Verification items for the finished model (mm, model axes). A direction names the side the tool comes from. Coordinates: 2 decimals unless noted, no trailing zeros. Loops run counter-clockwise (first coordinate to the right, second up) from the corner with the lowest first, then second, coordinate; pieces in that order, holes last. Notation, with made-up numbers: (-8.75, 37.5) - (5.25, 37.5) arc R19 ccw to (5.25, 72.5) - close; hole circle Ø8 at (68, 60.25). An arc over 180 degrees is marked (long way). One line per item, written item: value. Start each with the question number.
(1) Draft check along Z on faces 6 (the face through (18, -20, 0)), 7 (the face through (6, -64, 7)), 8 (the face through (16, -63, 0.3)), 9 (the face through (5, -69, 14)). Enter one of: +Z half, -Z half, draft (parallel to the pull), parting line (faces both ways), or undercut.
(2) Section check A-A (z = 14). Record the boundary of the cut face in (x, y).
(3) Set-up check for faces 1 (the face through (13.594, -40.048, 5.67)), 2 (the face through (5, -69, 4)), 3 (the face through (19, -21, 11.5)), 4 (the face through (9, -10, 6)), 5 (the face through (2.24, -10.52, 0.15)): record each of +Z, -Z, +X, -X, +Y, -Y from which the full face is reachable in a straight line by a thin tool's end or side.
(4) Section check C-C (z = 4). Record the boundary of the cut face in (x, y), plus the area to 3 significant figures.
(5) Section check D-D (y = -3.8). Record the boundary of the cut face in (x, z).
(6) Thickness scan on probe 1 along Z at (x, y) = (4, -70); probe 2 along Z at (x, y) = (1, 6.5); probe 3 along Y at (x, z) = (4.3, 14). Record the ranges inside material, lowest first. Write a range as [from, to].
(7) Section check B-B (x = 20.5). Record the boundary of the cut face in (y, z), plus the area to 3 significant figures.
(8) Gauge pin test, flat ends, axial feed: P1, Ø4, axis at y = 3.5, z = 4.5, coming from the -X side; P2, Ø9, axis at x = 14, z = 6.5, coming from the -Y side; P3, Ø12, axis at x = 9.5, y = -33.5, coming from the +Z side; P4, Ø7, axis at x = 2, y = -70, coming from the +Z side. Record the tip position at first contact, or that the pin passes through.
```python
from build123d import *

# Parameters (mm, degrees)
SKETCH003_R      = 5
SKETCH003_R_2    = 4.293562
SKETCH003_R_3    = 4.292919
SKETCH003_R_4    = 4.247298
SKETCH003_R_5    = 4.621938
SKETCH003_R_6    = 3.839764
EXTRUDE003_DEPTH = 0.3
SKETCH001_R      = 1
EXTRUDE001_DEPTH = 15
EXTRUDE_DEPTH    = 20
EXTRUDE002_DEPTH = 50


with BuildPart() as obj1:
    # Sketch003 → Extrude003 (new body)
    with BuildSketch(Plane.XY):
        with Locations((2.929235, 2.379341)):
            Circle(SKETCH003_R)
        with Locations((28.897633, 5.404075)):
            Circle(SKETCH003_R_2)
        with Locations((3.195543, -72.073357)):
            Circle(SKETCH003_R_3)
        with Locations((14.909943, -61.750763)):
            Circle(SKETCH003_R_4)
        with Locations((6.860642, -10.369777)):
            Circle(SKETCH003_R_5)
        with Locations((28.665668, -12.689456)):
            Circle(SKETCH003_R_6)
    extrude(amount=EXTRUDE003_DEPTH)


with BuildPart() as extrude001:
    # Sketch001 → Extrude001 (new body, symmetric)
    with BuildSketch(Plane.YZ):
        with Locations((-70, 4)):
            Circle(SKETCH001_R)
    extrude(amount=EXTRUDE001_DEPTH, both=True)


with BuildPart() as clone:
    # Clone base: copy of Extrude001
    add(extrude001.part)


with BuildPart() as clone_1:
    # Clone placement: moved
    add(clone.part.moved(Location((0, 0, 10))))


with BuildPart() as profil:
    # DWire → Extrude (new body)
    with BuildSketch(Plane.XY):
        with BuildLine():
            Line((10, -60), (17.29084, -19.529001))
            ThreePointArc((17.29084, -19.529001), (16.014131, -14.71074), (11.498558, -12.6))
            Line((11.498558, -12.6), (9, -12.6))
            Line((9, -12.6), (9, -7.6))
            Line((9, -7.6), (18.2, -7.6))
            ThreePointArc((18.2, -7.6), (22, -3.8), (18.2, 0))
            Line((18.2, 0), (3, 0))
            Line((3, 0), (3, 5))
            Line((3, 5), (29, 5))
            Line((29, 5), (29, -12.6))
            Line((29, -12.6), (15, -62))
            Line((15, -62), (5, -72))
            Line((5, -72), (3, -72))
            Line((3, -72), (3, -67))
            Line((3, -67), (10, -60))
        make_face()
    extrude(amount=EXTRUDE_DEPTH)


with BuildPart() as fusion:
    # Sketch002 → Extrude002 (new body, symmetric)
    with BuildSketch(Plane.YZ):
        Polygon((-83.421997, 18), (-67, 18), (-60.5, 11.5), (43.07156, 11.5), (44.937477, -15.860289), (-84.74369, -15.860289), align=None)
    extrude(amount=EXTRUDE002_DEPTH, both=True)

    # Common: intersect profil
    add(profil.part, mode=Mode.INTERSECT)

    # Cut: cut Clone
    add(clone_1.part, mode=Mode.SUBTRACT)

    # Cut001: cut Extrude001
    add(extrude001.part, mode=Mode.SUBTRACT)

    # Fusion: union obj1
    add(obj1.part)


solid = fusion.part
```
Responses:
1. face 6: -Z half
1. face 7: draft
1. face 8: +Z half
1. face 9: undercut
2. outline: (3, -72) - (5, -72) - (6, -71) - (3, -71) - close; (3, -69) - (8, -69) - (14, -63) - (7, -63) - (3, -67) - close
3. face 1: +Z, -Z, -X
3. face 2: +X, -X
3. face 3: +Z, +X, -X, +Y
3. face 4: +Z, -X
3. face 5: +Z, -Z
4. outline: (3, -72) - (5, -72) - (6, -71) - (3, -71) - close; (3, -69) - (8, -69) - (15, -62) - (29, -12.6) - (29, 5) - (3, 5) - (3, 0) - (18.2, 0) arc R3.8 cw to (18.2, -7.6) - (9, -7.6) - (9, -12.6) - (11.5, -12.6) arc R5.89 cw to (17.29, -19.53) - (10, -60) - (3, -67) - close
4. area: 742 mm²
5. outline: (22, 0) - (29, 0) - (29, 11.5) - (22, 11.5) - close
6. probe 1: z = [0, 3], [5, 13], [15, 18]
6. probe 2: z = [0, 0.3]
6. probe 3: y = [-72, -71], [-69, -65.7]
7. outline: (-42.59, 0) - (-6.82, 0) - (-6.82, 11.5) - (-42.59, 11.5) - close; (-0.78, 0) - (5, 0) - (5, 11.5) - (-0.78, 11.5) - close
7. area: 478 mm²
8. P1: stops at x = 3
8. P2: stops at y = -67.5
8. P3: stops at z = 11.5
8. P4: stops at z = 18
